```python
from build123d import *

# Parameters (mm, degrees)
SKETCH1_R           = 20
SKETCH1_R_2         = 10
SKETCH1_R_3         = 1.75
BOSS_EXTRUDE1_DEPTH = 4


with BuildPart() as part:
    # Sketch1 → Boss-Extrude1 (new body)
    with BuildSketch(Plane.XY):
        Circle(SKETCH1_R)
        Circle(SKETCH1_R_2, mode=Mode.SUBTRACT)
        with Locations((14.5, 0)):
            Circle(SKETCH1_R_3, mode=Mode.SUBTRACT)
        with Locations((-7.25, -12.557368355)):
            Circle(SKETCH1_R_3, mode=Mode.SUBTRACT)
        with Locations((-7.25, 12.557368355)):
            Circle(SKETCH1_R_3, mode=Mode.SUBTRACT)
    extrude(amount=BOSS_EXTRUDE1_DEPTH)


solid = part.part
```
For this review, take the finished solid that the model builds, in its own axes (mm). Round coordinates to 2 decimals unless told otherwise and drop trailing zeros. Write each loop counter-clockwise with the first axis right and the second up, starting at its lowest first coordinate (ties: lowest second). Pieces come first, ordered by that corner, then holes.
1) Insertion check: pin 1 Ø1 at (x, z) = (9.5, 0.5) entering from -Y; pin 2 Ø1.5 at (x, z) = (9, 1) entering from -Y; pin 3 Ø6 at (x, y) = (5.5, -10.5) entering from -Z; pin 4 Ø1.5 at (y, z) = (4, 1.5) entering from -X. Each pin has a flat end and moves straight along its axis. Give the tip position at first contact, or say it passes through.
Answer below:
pin 1: stops at y = -17.86
pin 2: stops at y = -18.22
pin 3: stops at z = 0
pin 4: stops at x = -19.73
2) Take a section at A-A on x = 0. Give the boundary of the cut face in (y, z).
Answer below:
outline: (-20, 0) - (-10, 0) - (-10, 4) - (-20, 4) - close; (10, 0) - (20, 0) - (20, 4) - (10, 4) - close
3) For line 1 along Y through (x, z) = (-7.25, 3.05); line 2 along Y through (x, z) = (0, 2.3); line 3 along X through (y, z) = (0.5, 0.25), list the stretches that pass through material, from the lowest coordinate up.
Answer below:
line 1: y = -18.64 to -14.31, -10.81 to -6.89, 6.89 to 10.81, 14.31 to 18.64
line 2: y = -20 to -10, 10 to 20
line 3: x = -19.99 to -9.99, 9.99 to 12.82, 16.18 to 19.99
4) Take a section at C-C on x = -7.25. Give the boundary of the cut face in (y, z), then the cut area to 3 significant figures.
Answer below:
outline: (-18.64, 0) - (-14.31, 0) - (-14.31, 4) - (-18.64, 4) - close; (-10.81, 0) - (-6.89, 0) - (-6.89, 4) - (-10.81, 4) - close; (6.89, 0) - (10.81, 0) - (10.81, 4) - (6.89, 4) - close; (14.31, 0) - (18.64, 0) - (18.64, 4) - (14.31, 4) - close
area: 66.0 mm2
5) Take a section at B-B on y = 0. Give the boundary of the cut face in (x, z), then the cut area to 3 significant figures.
Answer below:
outline: (-20, 0) - (-10, 0) - (-10, 4) - (-20, 4) - close; (10, 0) - (12.75, 0) - (12.75, 4) - (10, 4) - close; (16.25, 0) - (20, 0) - (20, 4) - (16.25, 4) - close
area: 66.0 mm2
6) Take a section at D-D on y = 7. Give the boundary of the cut face in (x, z) (3 decimals), then the cut area to 3 significant figures.
Answer below:
outline: (-18.735, 0) - (-7.141, 0) - (-7.141, 4) - (-18.735, 4) - close; (7.141, 0) - (18.735, 0) - (18.735, 4) - (7.141, 4) - close
area: 92.7 mm2
